from build123d import *

# Parameters (mm, degrees)
EXTRUDE_1_DEPTH     = 7
CUT_EXTRUDE_1_DEPTH = 4.25


with BuildPart() as part:
    # 草图1 → 凸台-拉伸1 (new body, symmetric)
    with BuildSketch(Plane.XY):
        with BuildLine():
            ThreePointArc((-3.083333333, 6.727039137), (0, -7.4), (3.083333333, 6.727039137))
            ThreePointArc((3.083333333, 6.727039137), (2.590940657, 8.052765147), (3.916666667, 8.545157823))
            ThreePointArc((3.916666667, 8.545157823), (0, -9.4), (-3.916666667, 8.545157823))
            ThreePointArc((-3.916666667, 8.545157823), (-2.590940657, 8.052765147), (-3.083333333, 6.727039137))
        make_face()
    extrude(amount=EXTRUDE_1_DEPTH, both=True)

    # 草图2 → 切除-拉伸1 (cut, symmetric)
    with BuildSketch(Plane.XY):
        with BuildLine():
            Line((-2.95212766, -6.785642363), (-3.75, -8.619599759))
            ThreePointArc((-3.75, -8.619599759), (-9.399556913, -0.091267984), (-3.916666667, 8.545157823))
            ThreePointArc((-3.916666667, 8.545157823), (-2.590940657, 8.052765147), (-3.083333333, 6.727039137))
            ThreePointArc((-3.083333333, 6.727039137), (-7.399651187, -0.071849264), (-2.95212766, -6.785642363))
        make_face()
        with BuildLine():
            Line((2.95212766, -6.785642363), (3.75, -8.619599759))
            ThreePointArc((3.75, -8.619599759), (9.399556913, -0.091267984), (3.916666667, 8.545157823))
            ThreePointArc((3.916666667, 8.545157823), (2.590940657, 8.052765147), (3.083333333, 6.727039137))
            ThreePointArc((3.083333333, 6.727039137), (7.399651187, -0.071849264), (2.95212766, -6.785642363))
        make_face()
    extrude(amount=CUT_EXTRUDE_1_DEPTH, both=True, mode=Mode.SUBTRACT)


solid = part.part
Can you work these out from the model? Positions are in its coordinate system, mm. A direction names the side the tool comes from. Round coordinates to 2 decimals unless told otherwise and drop trailing zeros. Loops run counter-clockwise (first coordinate to the right, second up) from the corner with the lowest first, then second, coordinate; pieces in that order, holes last. Notation, with made-up numbers: (-7.5, 20) - (41.5, 20) arc R13 cw to (41.5, 45) - close; hole circle Ø1 at (45.5, 43). An arc over 180 degrees is marked (long way). Use CSV: the item, a comma, the result in double quotes. Start each with the question number.
1) If we section it at A-A on y = 0: Write out the boundary of the cut face in (x, z), plus the area to 3 significant figures.
2) We'd pull the mould along Z, two halves only. Please class faces 4 (the cylindrical face through (-2.6, 8.07, 5.64)), 5 (the flat face through (0, -8, 7)), 6 (the flat face through (-8, 0, 4.25)): released by +Z, released by -Z, zero draft, split by the parting line, or undercut.
3) For pin 1 Ø1 at (x, z) = (-3.5, -0.5) entering from +Y; pin 2 Ø2 at (x, z) = (6, -5) entering from -Y; pin 3 Ø1 at (x, z) = (1.5, 2.5) entering from +Y, each with a flat end and sliding along its axis, tell me the tip position at first contact or that it passes through.
4) For faces 1 (the flat face through (0, -8, -7)), 2 (the flat face through (-3.345, -7.69, -0.059)), 3 (the flat face through (3.345, -7.69, 0.059)), which set-ups out of +Z, -Z, +X, -X, +Y, -Y let a thin tool reach every point of the face, with its end or its side?
5) If we section it at B-B on x = -4.25: Write out the boundary of the cut face in (y, z), plus the area to 3 significant figures.
6) Please list where these lines run through material, in increasing order: probe 1 along Z at (x, y) = (-7, 5); probe 2 along Y at (x, z) = (0, 3); probe 3 along X at (y, z) = (5.5, -5.5). Write a range as [from, to].
7) If we section it at C-C on x = 3.5: Write out the boundary of the cut face in (y, z).
8) If we section it at D-D on z = -3.5: Write out the boundary of the cut face in (x, y).
Geometry results:
1,outline,"(-9.4, -7) - (-7.4, -7) - (-7.4, -4.25) - (-9.4, -4.25) - close; (-9.4, 4.25) - (-7.4, 4.25) - (-7.4, 7) - (-9.4, 7) - close; (7.4, -7) - (9.4, -7) - (9.4, -4.25) - (7.4, -4.25) - close; (7.4, 4.25) - (9.4, 4.25) - (9.4, 7) - (7.4, 7) - close"
1,area,"22.0 mm2"
2,face 4,"zero draft"
2,face 5,"released by +Z"
2,face 6,"undercut"
3,pin 1,"stops at y = -6.9"
3,pin 2,"stops at y = -7.96"
3,pin 3,"stops at y = -7.12"
4,face 1,"-Z, +X, -X, +Y, -Y"
4,face 2,"-X, +Y"
4,face 3,"+X, +Y"
5,outline,"(-8.38, -7) - (-6.06, -7) - (-6.06, -4.25) - (-8.38, -4.25) - close; (-8.38, 4.25) - (-6.06, 4.25) - (-6.06, 7) - (-8.38, 7) - close; (6.06, -7) - (8.38, -7) - (8.38, -4.25) - (6.06, -4.25) - close; (6.06, 4.25) - (8.38, 4.25) - (8.38, 7) - (6.06, 7) - close"
5,area,"25.6 mm2"
6,probe 1,"z = [-7, -4.25], [4.25, 7]"
6,probe 2,"y = [-9.4, -7.4]"
6,probe 3,"x = [-7.62, -4.95], [4.95, 7.62]"
7,outline,"(-8.72, -7) - (-6.52, -7) - (-6.52, -4.25) - (-8.04, -4.25) - (-8.04, 4.25) - (-6.52, 4.25) - (-6.52, 7) - (-8.72, 7) - close; (6.52, -7) - (8.64, -7) - (8.64, -4.25) - (6.52, -4.25) - close; (6.52, 4.25) - (8.64, 4.25) - (8.64, 7) - (6.52, 7) - close"
8,outline,"(-3.75, -8.62) arc R9.4 ccw to (3.75, -8.62) - (2.95, -6.79) arc R7.4 cw to (-2.95, -6.79) - close"
